The model under review builds one solid part; all positions refer to its coordinate system, in mm. A direction names the side the tool comes from. Give positions to 0.01 mm unless a question says otherwise; leave off trailing zeros. Order: outer loops, then holes, each group sorted by start corner. A loop starts at its lowest first (then second) coordinate and runs counter-clockwise, first axis right, second up. Notation, with made-up numbers: (-37, 59) -> (8, 59) arc R6 cw to (8, 70) -> close; hole circle Ø3 at (23, 11.5). An arc over 180 degrees is marked (long way). Answer as a JSON object with one key per item and string values. Group by question number.
from build123d import *

# Parameters (mm, degrees)
BOSS_EXTRUDE1_START = 12.5
SKETCH2_R           = 2.5
BOSS_EXTRUDE1_DEPTH = 25
REVOLVE2_ANGLE      = 10
CIRPATTERN1_COUNT   = 15
CHAMFER1_SIZE       = 0.64


with BuildPart() as part:
    # Sketch2 → Boss-Extrude1 (new body)
    with BuildSketch(Plane(origin=(0, 0, 0), x_dir=(0, 0, -1), z_dir=(1, 0, 0)).offset(BOSS_EXTRUDE1_START)):
        Circle(SKETCH2_R)
    extrude(amount=-BOSS_EXTRUDE1_DEPTH)

    # Sketch5 → Revolve1 (revolve)
    with BuildSketch(Plane.XY, mode=Mode.PRIVATE) as revolve1_sk:
        with BuildLine():
            Line((-12.5, 0), (-12.5, 3.25))
            ThreePointArc((-12.5, 3.25), (-12.3, 3.45), (-12.1, 3.25))
            Line((-12.1, 3.25), (-12.1, 2.61341341))
            Line((-12.1, 2.61341341), (-11.202890026, 2.534926458))
            ThreePointArc((-11.202890026, 2.534926458), (-11.1, 2.5), (-11.024862675, 2.421510527))
            Line((-11.024862675, 2.421510527), (-9.626802921, 0))
            Line((-9.626802921, 0), (-12.5, 0))
        make_face()
    revolve(revolve1_sk.sketch.rotate(Axis((-12.5, 0, 0), (1, 0, 0)), 180), axis=Axis((-12.5, 0, 0), (1, 0, 0)))

    # Sketch6 → Revolve2 (revolve, symmetric)
    with BuildSketch(Plane.XY) as revolve2_sk:
        with BuildLine():
            Line((-12.1, 3.25), (-12.1, 0))
            Line((-12.1, 0), (-11.202890026, 0))
            Line((-11.202890026, 0), (-11.202890026, 2.534926458))
            ThreePointArc((-11.202890026, 2.534926458), (-11.264440532, 2.980844975), (-11.651445013, 3.210756524))
            Line((-11.651445013, 3.210756524), (-12.1, 3.25))
        make_face()
    revolve(axis=Axis((-12.1, 0, 0), (1, 0, 0)), revolution_arc=REVOLVE2_ANGLE / 2)
    revolve(revolve2_sk.sketch, axis=Axis((-12.1, 0, 0), (-1, 0, 0)), revolution_arc=REVOLVE2_ANGLE / 2)

    # CirPattern1: part ×15 about axis
    cirpattern1_axis = Axis((0, 0, 0), (1, 0, 0))


with BuildPart() as part_1:
    add(part.part)
    for i in range(1, CIRPATTERN1_COUNT):
        add(part.part.rotate(cirpattern1_axis, i * 360 / CIRPATTERN1_COUNT))

    # Chamfer1
    chamfer1_edges = [part_1.edges().sort_by_distance(p)[0] for p in [
        (12.5, 0, 2.5),
    ]]
    chamfer(chamfer1_edges, length=CHAMFER1_SIZE)


solid = part_1.part
1. Take a section at B-B on x = 6. Give the boundary of the cut face in (y, z).
2. Draft analysis for pull direction Z (two halves, no side actions). For faces 3 (the flat face through (12.5, 0, 0)), 4 (the cylindrical face through (0.54, -2.44, 0.54)), 5 (the flat face through (-12.1, -2, -2)), state which applies: pulls with the +Z half, pulls with the -Z half, needs draft (parallel to the pull), parting line crosses it, or undercut.
3. For pin 1 (0.8 mm diameter, centred on y = 0.5, z = -3, fed in from +X); pin 2 (2 mm diameter, centred on x = -7.5, z = -2.5, fed in from -Y); pin 3 (2 mm diameter, centred on x = -8, y = 1.5, fed in from +Z), all flat-tipped, find the tip position at first contact; note any pin that passes through.
4. Machinability: for faces 1 (the flat face through (-12.5, 0, 0)), 2 (the flat face through (-12.1, -2.7, -1.2)), which of the approach directions +Z, -Z, +X, -X, +Y, -Y give a long, thin tool a straight path to every point of the face, cutting with its end or side? Answer none if there is none.
5. Take a section at A-A on z = 0. Give the boundary of the cut face in (x, y).
6. For probe 1 along Y at (x, z) = (2.25, -1); probe 2 along Y at (x, z) = (1.5, 0); probe 3 along Z at (x, y) = (-4.5, 0.25), list the stretches that pass through material, from the lowest coordinate up. Write a range as [from, to].
Checks:
{
 "1": {"outline": "circle Ø5 at (0, 0)"},
 "2": {"face 3": "needs draft", "face 4": "parting line crosses it", "face 5": "undercut"},
 "3": {"pin 1": "stops at x = -11.18", "pin 2": "stops at y = -2", "pin 3": "stops at z = 2.45"},
 "4": {"face 1": "+Z, -Z, -X, +Y, -Y", "face 2": "+X"},
 "5": {"outline": "(-12.5, -3.25) arc R0.2 ccw to (-12.1, -3.25) -> (-12.1, -2.61) -> (-11.2, -2.53) arc R0.23 ccw to (-11.1, -2.5) -> (11.86, -2.5) -> (12.5, -1.86) -> (12.5, 1.86) -> (11.86, 2.5) -> (-11.1, 2.5) arc R0.23 ccw to (-11.2, 2.53) arc R0.52 ccw to (-11.65, 3.21) -> (-12.1, 3.25) arc R0.2 ccw to (-12.5, 3.25) -> close"},
 "6": {"probe 1": "y = [-2.29, 2.29]", "probe 2": "y = [-2.5, 2.5]", "probe 3": "z = [-2.49, 2.49]"}
}
